```python
from build123d import *

# Parameters (mm, degrees)
SKETCH1_W           = 16
SKETCH1_H           = 114
BOSS_EXTRUDE2_DEPTH = 2
SKETCH2_W           = 16
SKETCH2_H           = 2
BOSS_EXTRUDE3_DEPTH = 20
SKETCH3_W           = 16
SKETCH3_H           = 2
BOSS_EXTRUDE4_DEPTH = 20
SKETCH4_R           = 2
CUT_EXTRUDE2_DEPTH  = 118.247641795


with BuildPart() as part:
    # Sketch1 → Boss-Extrude2 (new body)
    with BuildSketch(Plane.XY):
        with Locations((8.340425532, 57.170212766)):
            Rectangle(SKETCH1_W, SKETCH1_H)
    extrude(amount=BOSS_EXTRUDE2_DEPTH)

    # Sketch2 → Boss-Extrude3 (add)
    with BuildSketch(Plane.XY.offset(2)):
        with Locations((8.340425532, 113.170212766)):
            Rectangle(SKETCH2_W, SKETCH2_H)
    extrude(amount=BOSS_EXTRUDE3_DEPTH)

    # Sketch3 → Boss-Extrude4 (add)
    with BuildSketch(Plane.XY.offset(2)):
        with Locations((8.340425532, 1.170212766)):
            Rectangle(SKETCH3_W, SKETCH3_H)
    extrude(amount=BOSS_EXTRUDE4_DEPTH)

    # Sketch4 → Cut-Extrude2 (cut, through all)
    with BuildSketch(Plane(origin=(0, 114.170212766, 0), x_dir=(1, 0, 0), z_dir=(0, 1, 0))):
        with Locations(Location((8.340425532, -10, 0), (0, 0, 270))):
            Circle(SKETCH4_R)
    extrude(amount=-CUT_EXTRUDE2_DEPTH, mode=Mode.SUBTRACT)


solid = part.part
```
Build history of the part. All positions in model axes, mm. A direction names the side the tool comes from. Give positions to 0.01 mm unless a question says otherwise; leave off trailing zeros. Loops run counter-clockwise (first coordinate to the right, second up) from the corner with the lowest first, then second, coordinate; pieces in that order, holes last.
1) Probe line 1 along Y through (x, z) = (10.5, 17.5); line 2 along X through (y, z) = (112.9, 10); line 3 along Z through (x, y) = (6.5, 91). List the from-to ranges inside material, lowest first.
Values follow:
line 1: y = 0.17 to 2.17, 112.17 to 114.17
line 2: x = 0.34 to 6.34, 10.34 to 16.34
line 3: z = 0 to 2
2) 3-axis set-ups, long thin cutter, end or side, ignore diameter. For faces 1 (the face through (10, 112.17, 12)), 2 (the face through (6, 0.17, 11)): which of +Z, -Z, +X, -X, +Y, -Y reach the whole face in a straight line?
Values follow:
face 1: +Z, +X, -X
face 2: +Z, -Z, +X, -X, -Y
3) Two-plate mould, pull along X, no slides. Class faces 3 (the face through (7.123, 113.184, 8.413)), 4 (the face through (16.34, 44.2, 0.4)), 5 (the face through (6, 114.17, 11)), 6 (the face through (0.34, 44.2, 0.4)): released by +X, released by -X, zero draft, split by the parting line, or undercut.
Values follow:
face 3: undercut
face 4: released by +X
face 5: zero draft
face 6: released by -X
4) Drop flat-ended pins along their axis: P1, Ø1, axis at x = 12.5, y = 52.5, coming from the +Z side; P2, Ø4.5, axis at x = 8.34, z = 10, coming from the +Y side. Give the stop position or say it passes through.
Values follow:
P1: stops at z = 2
P2: stops at y = 114.17
5) Band-saw the part on A-A on z = 17.75. List the corners of the cut face in (x, y).
Values follow:
outline: (0.34, 0.17) - (16.34, 0.17) - (16.34, 2.17) - (0.34, 2.17) - close; (0.34, 112.17) - (16.34, 112.17) - (16.34, 114.17) - (0.34, 114.17) - close
6) Band-saw the part on B-B on z = 10. List the corners of the cut face in (x, y), then the cut area to 3 significant figures.
Values follow:
outline: (0.34, 0.17) - (6.34, 0.17) - (6.34, 2.17) - (0.34, 2.17) - close; (0.34, 112.17) - (6.34, 112.17) - (6.34, 114.17) - (0.34, 114.17) - close; (10.34, 0.17) - (16.34, 0.17) - (16.34, 2.17) - (10.34, 2.17) - close; (10.34, 112.17) - (16.34, 112.17) - (16.34, 114.17) - (10.34, 114.17) - close
area: 48.0 mm2
7) Band-saw the part on C-C on x = 14.25. List the corners of the cut face in (y, z), then the cut area to 3 significant figures.
Values follow:
outline: (0.17, 0) - (114.17, 0) - (114.17, 22) - (112.17, 22) - (112.17, 2) - (2.17, 2) - (2.17, 22) - (0.17, 22) - close
area: 308 mm2
8) Band-saw the part on D-D on y = 16.5. List the corners of the cut face in (x, z).
Values follow:
outline: (0.34, 0) - (16.34, 0) - (16.34, 2) - (0.34, 2) - close
